Verification items for the finished model (mm, model axes). A direction names the side the tool comes from. Give positions to 0.01 mm unless a question says otherwise; leave off trailing zeros. Loops run counter-clockwise (first coordinate to the right, second up) from the corner with the lowest first, then second, coordinate; pieces in that order, holes last. Notation, with made-up numbers: (2, -35.5) -> (60, -35.5) arc R20 ccw to (60, -11.5) -> close; hole circle Ø6 at (86, -21.75). An arc over 180 degrees is marked (long way). Use one line per item in the form item = value. Start each with the question number.
from build123d import *

# Parameters (mm, degrees)
SKETCH1_R           = 6.25
BOSS_EXTRUDE1_DEPTH = 125
SKETCH3_R           = 6.25
BOSS_EXTRUDE2_DEPTH = 10
SKETCH6_R           = 6.25
BOSS_EXTRUDE3_DEPTH = 10
SKETCH8_R           = 6.25
BOSS_EXTRUDE4_DEPTH = 10
SKETCH9_R           = 6.25
BOSS_EXTRUDE6_DEPTH = 10
SKETCH14_R          = 6.25
BOSS_EXTRUDE7_DEPTH = 25


with BuildPart() as part:
    # Sketch1 → Boss-Extrude1 (new body)
    with BuildSketch(Plane.XY):
        Circle(SKETCH1_R)
    extrude(amount=BOSS_EXTRUDE1_DEPTH)

    # Sketch3 → Boss-Extrude2 (add)
    with BuildSketch(Plane(origin=(0, 0, 15), x_dir=(-1, 0, 0), z_dir=(0, 0, -1))):
        with BuildLine():
            Line((-2.443849423, 11.74), (-7.168624973, 5.104))
            ThreePointArc((-7.168624973, 5.104), (0, -8.8), (7.168624973, 5.104))
            Line((7.168624973, 5.104), (2.443849423, 11.74))
            ThreePointArc((2.443849423, 11.74), (0, 13), (-2.443849423, 11.74))
        make_face()
        Circle(SKETCH3_R, mode=Mode.SUBTRACT)
    extrude(amount=-BOSS_EXTRUDE2_DEPTH)

    # Sketch6 → Boss-Extrude3 (add)
    with BuildSketch(Plane(origin=(0, 0, 40), x_dir=(-1, 0, 0), z_dir=(0, 0, -1))):
        with BuildLine():
            Line((-2.443849423, -11.74), (-7.168624973, -5.104))
            ThreePointArc((-7.168624973, -5.104), (0, 8.8), (7.168624973, -5.104))
            Line((7.168624973, -5.104), (2.443849423, -11.74))
            ThreePointArc((2.443849423, -11.74), (0, -13), (-2.443849423, -11.74))
        make_face()
        Circle(SKETCH6_R, mode=Mode.SUBTRACT)
    extrude(amount=-BOSS_EXTRUDE3_DEPTH)

    # Sketch8 → Boss-Extrude4 (add)
    with BuildSketch(Plane(origin=(0, 0, 90), x_dir=(-1, 0, 0), z_dir=(0, 0, -1))):
        with BuildLine():
            ThreePointArc((2.443849423, 11.74), (0, 13), (-2.443849423, 11.74))
            Line((-2.443849423, 11.74), (-2.456936947, 11.721470546))
            Line((-2.456936947, 11.721470546), (-6.737843427, 5.66051817))
            Line((-6.737843427, 5.66051817), (-7.587481927, 4.457591055))
            ThreePointArc((-7.587481927, 4.457591055), (0.385125198, -8.791568608), (7.168624973, 5.104))
            Line((7.168624973, 5.104), (2.443849423, 11.74))
        make_face()
        Circle(SKETCH8_R, mode=Mode.SUBTRACT)
    extrude(amount=-BOSS_EXTRUDE4_DEPTH)

    # Sketch9 → Boss-Extrude6 (add)
    with BuildSketch(Plane(origin=(0, 0, 115), x_dir=(-1, 0, 0), z_dir=(0, 0, -1))):
        with BuildLine():
            Line((2.443849423, -11.74), (7.168624973, -5.104))
            ThreePointArc((7.168624973, -5.104), (0, 8.8), (-7.168624973, -5.104))
            Line((-7.168624973, -5.104), (-2.443849423, -11.74))
            ThreePointArc((-2.443849423, -11.74), (0, -13), (2.443849423, -11.74))
        make_face()
        Circle(SKETCH9_R, mode=Mode.SUBTRACT)
    extrude(amount=-BOSS_EXTRUDE6_DEPTH)

    # Sketch14 → Boss-Extrude7 (add)
    with BuildSketch(Plane.XY.offset(125)):
        Circle(SKETCH14_R)
    extrude(amount=BOSS_EXTRUDE7_DEPTH)


solid = part.part
Item 1: Material ranges on line 1 (Z direction, x = 4.25, y = -6); line 2 (Z direction, x = -5.25, y = -7.25); line 3 (Y direction, x = 2.5, z = 141), recorded low to high.
Item 2: Sectioned sample at B-B, the plane z = 95.5. Enter the section's corners in (x, y), and give its area (3 significant figures).
Item 3: Sectioned sample at A-A, the plane y = 7.5. Enter the section's corners in (x, z).
Item 4: Sectioned sample at D-D, the plane z = 20.5. Enter the section's corners in (x, y).
Item 5: Gauge pin test, flat ends, axial feed: pin 1 Ø8 at (x, z) = (-0.5, 58) entering from -Y; pin 2 Ø2 at (x, z) = (5.5, 30) entering from +Y; pin 3 Ø10 at (x, z) = (-6.5, 45.5) entering from -Y. Record the tip position at first contact, or that the pin passes through.
Item 6: Sectioned sample at C-C, the plane z = 112. Enter the section's corners in (x, y).
Item 7: Tool access check on faces 1 (the cylindrical face through (-0.1, -8.8, 94.9)), 2 (the cylindrical face through (5.96, 1.88, 7.4)), 3 (the flat face through (0, -7, 125)). Record the directions out of +Z, -Z, +X, -X, +Y, -Y that give a thin tool (end or side, any length) a straight path to the whole face; none if there is none.
Item 8: Draft check along Z on faces 4 (the flat face through (4.77, 8.47, 19.93)), 5 (the flat face through (0, 0, 150)), 6 (the cylindrical face through (5.96, 1.88, 107.4)). Enter one of: +Z half, -Z half, draft (parallel to the pull), parting line (faces both ways), or undercut.
Outcome:
q1.line_1 = 15 to 25, 40 to 50, 90 to 100, 115 to 125
q1.line_2 = 40 to 50, 115 to 125
q1.line_3 = -5.73 to 5.73
q2.outline = (-7.17, 5.1) arc R8.8 ccw (long way) to (7.59, 4.46) -> (2.44, 11.74) arc R3 ccw to (-2.44, 11.74) -> close
q2.area = 274 mm^2
q3.outline = (-5.46, 15) -> (5.46, 15) -> (5.46, 25) -> (-5.46, 25) -> close; (-5.46, 90) -> (5.44, 90) -> (5.44, 100) -> (-5.46, 100) -> close; (-4.6, 40) -> (4.6, 40) -> (4.6, 50) -> (-4.6, 50) -> close; (-4.6, 115) -> (4.6, 115) -> (4.6, 125) -> (-4.6, 125) -> close
q4.outline = (-7.17, 5.1) arc R8.8 ccw (long way) to (7.17, 5.1) -> (2.44, 11.74) arc R3 ccw to (-2.44, 11.74) -> close
q5.pin_1 = -6.25
q5.pin_2 = 4.34
q5.pin_3 = -12.6
q6.outline = circle Ø12.5 at (0, 0)
q7.face_1 = none
q7.face_2 = -Z
q7.face_3 = +Z
q8.face_4 = draft
q8.face_5 = +Z half
q8.face_6 = undercut
